from build123d import *

# Parameters (mm, degrees)
SALIENTE_EXTRUIR1_DEPTH = 15
REDONDEO1_R             = 2
CROQUIS2_R              = 2.5
CORTAR_EXTRUIR1_DEPTH   = 73


# Read off the part's stored shape, not the designer's step: Saliente-Extruir1
with BuildPart() as part:
    # Saliente-Extruir1 outline → Saliente-Extruir1 (new body)
    with BuildSketch(Plane(origin=(0, 0, 0), x_dir=(1, 0, 0), z_dir=(0, 1, 0))):
        with BuildLine():
            Line((33.547312235, 9.5), (33.547312235, 14.5))
            Line((33.547312235, 14.5), (21.581241855, 14.5))
            ThreePointArc((21.581241855, 14.5), (-26, 0), (21.581241855, -14.5))
            Line((21.581241855, -14.5), (33.547312235, -14.5))
            Line((33.547312235, -14.5), (33.547312235, -9.5))
            Line((33.547312235, -9.5), (20.396078054, -9.5))
            ThreePointArc((20.396078054, -9.5), (-22.5, 0), (20.396078054, 9.5))
            Line((20.396078054, 9.5), (33.547312235, 9.5))
        make_face()
    extrude(amount=SALIENTE_EXTRUIR1_DEPTH)

    # Redondeo1
    redondeo1_edges = [part.edges().sort_by_distance(p)[0] for p in [
        (-26, 0, 0),
        (33.547312235, 0, -12),
        (-26, 15, 0),
        (33.547312235, 15, 12),
        (33.547312235, 15, -12),
        (33.547312235, 0, 12),
    ]]
    fillet(redondeo1_edges, radius=REDONDEO1_R)

    # Croquis2 → Cortar-Extruir1 (cut)
    with BuildSketch(Plane.XY.offset(14.5)):
        with Locations((27.564277045, 7.5)):
            Circle(CROQUIS2_R)
    extrude(amount=-CORTAR_EXTRUIR1_DEPTH, mode=Mode.SUBTRACT)


solid = part.part
Here's how the part is built. I have some questions about the finished solid (model axes, mm). A direction names the side the tool comes from. Round coordinates to 2 decimals unless told otherwise and drop trailing zeros. Write each loop counter-clockwise with the first axis right and the second up, starting at its lowest first coordinate (ties: lowest second). Pieces come first, ordered by that corner, then holes. Notation, with made-up numbers: (70, 14) -> (101, 14) arc R6 ccw to (101, 21) -> close; hole circle Ø7 at (33, 53.5). An arc over 180 degrees is marked (long way). One line per item, written item: value.
1) Suppose I cut it at B-B on z = 0. List the corners of the cut face in (x, y) for me, plus the area to 3 significant figures.
Filled sheet:
outline: (-26, 2) arc R2 ccw to (-24, 0) -> (-22.5, 0) -> (-22.5, 15) -> (-24, 15) arc R2 ccw to (-26, 13) -> close
area: 50.8 mm2
2) Suppose I cut it at C-C on y = 3.5. List the corners of the cut face in (x, z) for me.
Filled sheet:
outline: (20.4, -9.5) arc R22.5 cw (long way) to (20.4, 9.5) -> (33.55, 9.5) -> (33.55, 14.5) -> (21.58, 14.5) arc R26 ccw (long way) to (21.58, -14.5) -> (33.55, -14.5) -> (33.55, -9.5) -> close
3) If I drill on line 1 (Z direction, x = 25, y = 9.75); line 2 (Z direction, x = -20, y = 7.5); line 3 (X direction, y = 0.5, z = -11.5), over which ranges is the centre line in solid material (lowest first)? Write a range as [from, to].
Filled sheet:
line 1: z = [-14.5, -9.5], [9.5, 14.5]
line 2: z = [-16.61, -10.31], [10.31, 16.61]
line 3: x = [-22.56, -19.34], [19.34, 32.87]
4) Suppose I cut it at A-A on y = 7.5. List the corners of the cut face in (x, z) for me.
Filled sheet:
outline: (20.4, -9.5) arc R22.5 cw (long way) to (20.4, 9.5) -> (25.06, 9.5) -> (25.06, 14.5) -> (21.58, 14.5) arc R26 ccw (long way) to (21.58, -14.5) -> (25.06, -14.5) -> (25.06, -9.5) -> close; (30.06, -14.5) -> (33.55, -14.5) -> (33.55, -9.5) -> (30.06, -9.5) -> close; (30.06, 9.5) -> (33.55, 9.5) -> (33.55, 14.5) -> (30.06, 14.5) -> close
5) For faces 1 (the face through (-22.484, 7.395, 0.852)), 2 (the face through (25, 9, -9.5)), which set-ups out of +Z, -Z, +X, -X, +Y, -Y let a thin tool reach every point of the face, with its end or its side?
Filled sheet:
face 1: +Y, -Y
face 2: +X, +Y, -Y
6) We'd pull the mould along X, two halves only. Please class faces 3 (the face through (25.58, 5.98, 12.04)), 4 (the face through (32.977, 0.601, 11.965)), 5 (the face through (20, 15, 11)), 6 (the face through (25.58, 5.98, -11.96)): released by +X, released by -X, zero draft, split by the parting line, or undercut.
Filled sheet:
face 3: undercut
face 4: released by +X
face 5: zero draft
face 6: undercut
7) I'm going to push flat-ended pins straight in: pin 1 Ø3 at (x, y) = (2.5, 8.5) entering from +Z; pin 2 Ø4.5 at (x, y) = (24.5, 8.5) entering from -Z; pin 3 Ø6 at (x, y) = (27.56, 7.5) entering from +Z. Where does each tip first touch, or does it pass through?
Filled sheet:
pin 1: stops at z = 25.98
pin 2: stops at z = -14.5
pin 3: stops at z = 14.5
